Verification items for the finished model (mm, model axes). Face numbers are marked on the shaded views. A direction names the side the tool comes from. Give positions to 0.01 mm unless a question says otherwise; leave off trailing zeros. Order: outer loops, then holes, each group sorted by start corner. A loop starts at its lowest first (then second) coordinate and runs counter-clockwise, first axis right, second up. Notation, with made-up numbers: (38, 7.5) - (96, 7.5) arc R28 cw to (96, 29.5) - close; hole circle Ø6 at (72.5, 78). An arc over 180 degrees is marked (long way). Answer as a JSON object with one key per item and string values. Group by question number.
(1) Section check A-A (y = 2.25). Record the boundary of the cut face in (x, z).
(2) Section check B-B (y = -2.75). Record the boundary of the cut face in (x, z), then the cut area to 3 significant figures.
(3) Depth check by flat-ended pin: pin 1 Ø1 at (y, z) = (3, 2.5) entering from +X; pin 2 Ø1 at (x, y) = (-2.5, -2) entering from -Z; pin 3 Ø1.5 at (y, z) = (-2, -2.5) entering from +X. Enter the tip coordinate at first touch or a pass-through.
(4) Mould release check, pull along X, two halves, no side actions. Record for the marked faces 4, 5 and 6: +X half, -X half, draft (parallel to the pull), parting line (faces both ways), or undercut.
(5) Thickness scan on line 1 (X direction, y = 2.25, z = 0); line 2 (Y direction, x = 1.75, z = -5.25); line 3 (X direction, y = 2.5, z = -2.5). Record the ranges inside material, lowest first.
(6) Access from +Z, -Z, +X, -X, +Y, -Y to the whole of each face (thin tool, end or side, straight path). Record for the marked faces 1, 2 and 3.
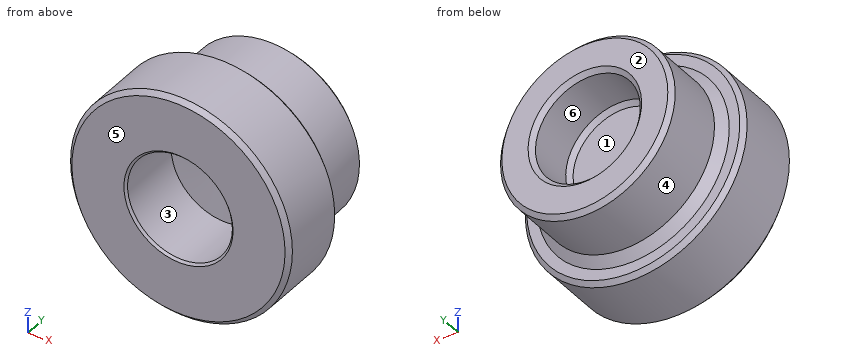
```python
from build123d import *

# Parameters (mm, degrees)
SKETCH1_R                       = 5
SKETCH1_R_2                     = 3
BOSS_EXTRUDE1_DEPTH             = 1
SKETCH1_3_R                     = 5
SKETCH1_3_R_2                   = 3
BOSS_EXTRUDE2_DEPTH             = 4
CHAMFER1_SIZE                   = 0.25
SKETCH5_R                       = 6.35
BOSS_EXTRUDE4_DEPTH             = 4
F_6_0MM_DOWEL_HOLE1_D           = 6
F_6_0MM_DOWEL_HOLE1_DEPTH       = 3.737534009
F_6_0MM_DOWEL_HOLE1_CSINK_D     = 6.25
F_6_0MM_DOWEL_HOLE1_CSINK_ANGLE = 90
F_6_0MM_DOWEL_HOLE1_TIP         = 0.262465991
CHAMFER2_SIZE                   = 0.25
CHAMFER3_SIZE                   = 0.5


with BuildPart() as part:
    # Sketch1 → Boss-Extrude1 (new body)
    with BuildSketch(Plane(origin=(0, 0, 0), x_dir=(1, 0, 0), z_dir=(0, 1, 0))):
        with Locations(Location((0, 0, 0), (0, 0, 270))):
            Circle(SKETCH1_R)
        Circle(SKETCH1_R_2, mode=Mode.SUBTRACT)
        Circle(SKETCH1_R_2)
    extrude(amount=BOSS_EXTRUDE1_DEPTH)

    # Sketch1_3 → Boss-Extrude2 (add)
    with BuildSketch(Plane(origin=(0, 0, 0), x_dir=(1, 0, 0), z_dir=(0, 1, 0))):
        with Locations(Location((0, 0, 0), (0, 0, 270))):
            Circle(SKETCH1_3_R)
        with Locations(Location((0, 0, 0), (0, 0, 270))):
            Circle(SKETCH1_3_R_2, mode=Mode.SUBTRACT)
    extrude(amount=BOSS_EXTRUDE2_DEPTH)

    # Chamfer1
    chamfer1_edges = [part.edges().sort_by_distance(p)[0] for p in [
        (0, 1, -3),
        (0, 4, -5),
        (0, 4, -3),
    ]]
    chamfer(chamfer1_edges, length=CHAMFER1_SIZE)

    # Sketch5 → Boss-Extrude4 (add)
    with BuildSketch(Plane(origin=(0, 0, 0), x_dir=(1, 0, 0), z_dir=(0, 1, 0))):
        with Locations(Location((0, 0, 0), (0, 0, 270))):
            Circle(SKETCH5_R)
    extrude(amount=-BOSS_EXTRUDE4_DEPTH)

    # 6.0mm Dowel Hole1
    with Locations(Plane(origin=(0, -4, 0), x_dir=(-1, 0, 0), z_dir=(0, -1, 0))):
        with Locations((0, 0)):
            CounterSinkHole(F_6_0MM_DOWEL_HOLE1_D / 2, F_6_0MM_DOWEL_HOLE1_CSINK_D / 2, depth=F_6_0MM_DOWEL_HOLE1_DEPTH, counter_sink_angle=F_6_0MM_DOWEL_HOLE1_CSINK_ANGLE)
            with Locations((0, 0, -(F_6_0MM_DOWEL_HOLE1_DEPTH + F_6_0MM_DOWEL_HOLE1_TIP / 2))):  # 170° drill point
                Cone(0, F_6_0MM_DOWEL_HOLE1_D / 2, F_6_0MM_DOWEL_HOLE1_TIP, mode=Mode.SUBTRACT)

    # Chamfer2
    chamfer2_edges = [part.edges().sort_by_distance(p)[0] for p in [
        (0, -4, -6.35),
        (0, 0, -6.35),
    ]]
    chamfer(chamfer2_edges, length=CHAMFER2_SIZE)

    # Chamfer3
    chamfer3_edges = [part.edges().sort_by_distance(p)[0] for p in [
        (0, 0, -5),
    ]]
    chamfer(chamfer3_edges, length=CHAMFER3_SIZE)


solid = part.part
```
Solutions:
{
 "1": {"outline": "circle Ø10 at (0, 0); hole circle Ø6 at (0, 0)"},
 "2": {"outline": "circle Ø12.7 at (0, 0); hole circle Ø6 at (0, 0)", "area": "98.4 mm2"},
 "3": {"pin 1": "stops at x = 4.58", "pin 2": "stops at z = -6.03", "pin 3": "stops at x = 6.1"},
 "4": {"face 4": "parting line", "face 5": "draft", "face 6": "undercut"},
 "5": {"line 1": "x = -5 to -3, 3 to 5", "line 2": "y = -4 to 0", "line 3": "x = -4.33 to -1.66, 1.66 to 4.33"},
 "6": {"face 1": "+Y", "face 2": "+Z, -Z, +X, -X, +Y", "face 3": "-Y"}
}
